CAD build for the part. Positions are in the model's coordinates, mm. Coordinates: 2 decimals unless noted, no trailing zeros. Write each loop counter-clockwise with the first axis right and the second up, starting at its lowest first coordinate (ties: lowest second). Pieces come first, ordered by that corner, then holes. Notation, with made-up numbers: M -16.75,58.5 L 42.25,58.5 A18 cw 42.25,83.5 Z; hole C 69,-31 d11. An arc over 180 degrees is marked long. Answer as CSV lines item,"result". Start each with the question number.
```python
from build123d import *
from build123d.topology import SkipClean

# Parameters (mm, degrees)
BOSS_EXTRUDE1_DEPTH = 5
SKETCH2_R           = 2.525
CUT_EXTRUDE1_DEPTH  = 2
SKETCH3_R           = 4
BOSS_EXTRUDE2_DEPTH = 30


with BuildPart() as part:
    # Sketch1 → Boss-Extrude1 (new body)
    with BuildSketch(Plane(origin=(0, 0, 0), x_dir=(1, 0, 0), z_dir=(0, 1, 0))):
        with BuildLine():
            Line((0, 0), (39, 0))
            ThreePointArc((39, 0), (43.000000182, -3.999999909), (39.000000182, -8))
            Line((39.000000182, -8), (1.82e-07, -8))
            ThreePointArc((1.82e-07, -8), (-4, -4.000000091), (0, 0))
        make_face()
    extrude(amount=BOSS_EXTRUDE1_DEPTH)

    # Sketch2 → Cut-Extrude1 (cut)
    with BuildSketch(Plane(origin=(0, 0, 0), x_dir=(1, 0, 0), z_dir=(0, 1, 0))):
        with Locations(Location((0, -4, 0), (0, 0, 270))):
            Circle(SKETCH2_R)
    extrude(amount=CUT_EXTRUDE1_DEPTH, mode=Mode.SUBTRACT)

    # Sketch3 → Boss-Extrude2 (add)
    with SkipClean():  # the faces are left unmerged after this step: merging them gives an invalid solid
        with BuildSketch(Plane(origin=(0, 0, 0), x_dir=(1, 0, 0), z_dir=(0, 1, 0))):
            with Locations(Location((39.000000182, -4, 0), (0, 0, 270))):
                Circle(SKETCH3_R)
        extrude(amount=BOSS_EXTRUDE2_DEPTH)


solid = part.part
```
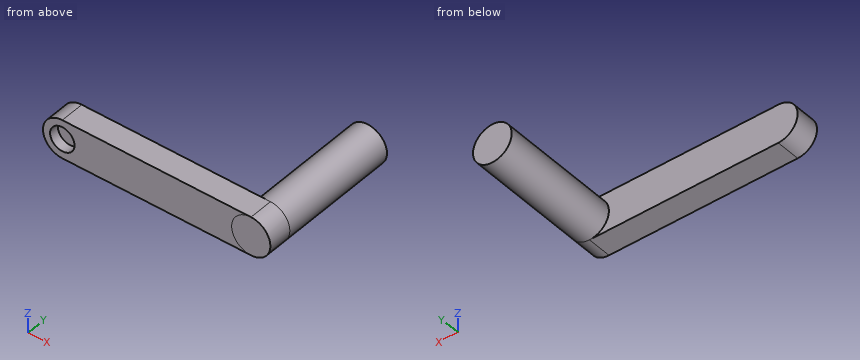
1) Pin check, flat tips, straight feed: P1, Ø1, axis at x = 36.5, y = 26.5, coming from the +Z side; P2, Ø2.5, axis at x = 20.5, z = 4.5, coming from the +Y side; P3, Ø3, axis at y = 20.5, z = 4, coming from the -X side. Stop position of each tip, or through.
2) Band-saw the part on A-A, the plane z = 4. List the corners of the cut face in (x, y) (3 decimals), plus the area to 3 significant figures.
3) Band-saw the part on C-C, the plane y = 13. List the corners of the cut face in (x, z).
4) Band-saw the part on B-B, the plane x = 3. List the corners of the cut face in (y, z).
5) Probe L1, parallel to X at y = 0.65, z = 4 (3 decimals); L2, parallel to Y at x = 11.5, z = 1; L3, parallel to X at y = 16.25, z = 4. List the from-to ranges inside material, lowest first. Write a range as [from, to].
Result sheet:
1,P1,"stops at z = 7.46"
1,P2,"stops at y = 5"
1,P3,"stops at x = 35"
2,outline,"M -4,0 L -2.525,0 L -2.525,2 L 2.525,2 L 2.525,0 L 43,0 L 43,30 L 35,30 L 35,5 L -4,5 Z"
2,area,"425 mm²"
3,outline,"C 39,4 d8"
4,outline,"M 0,0 L 5,0 L 5,8 L 0,8 Z"
5,L1,"x = [-4, -2.525], [2.525, 43]"
5,L2,"y = [0, 5]"
5,L3,"x = [35, 43]"
